Source: three-view drawing plus pictorial views. Frame: mm from the lowest corner of the part. Round coordinates to 2 decimals unless told otherwise and drop trailing zeros. Loops run counter-clockwise (first coordinate to the right, second up) from the corner with the lowest first, then second, coordinate; pieces in that order, holes last. Notation, with made-up numbers: M 73,-12 L 124,-12 A21 ccw 124,25 Z; hole C -37.5,56 d2. An arc over 180 degrees is marked long. Answer as a JSON object with one key per item and string values.
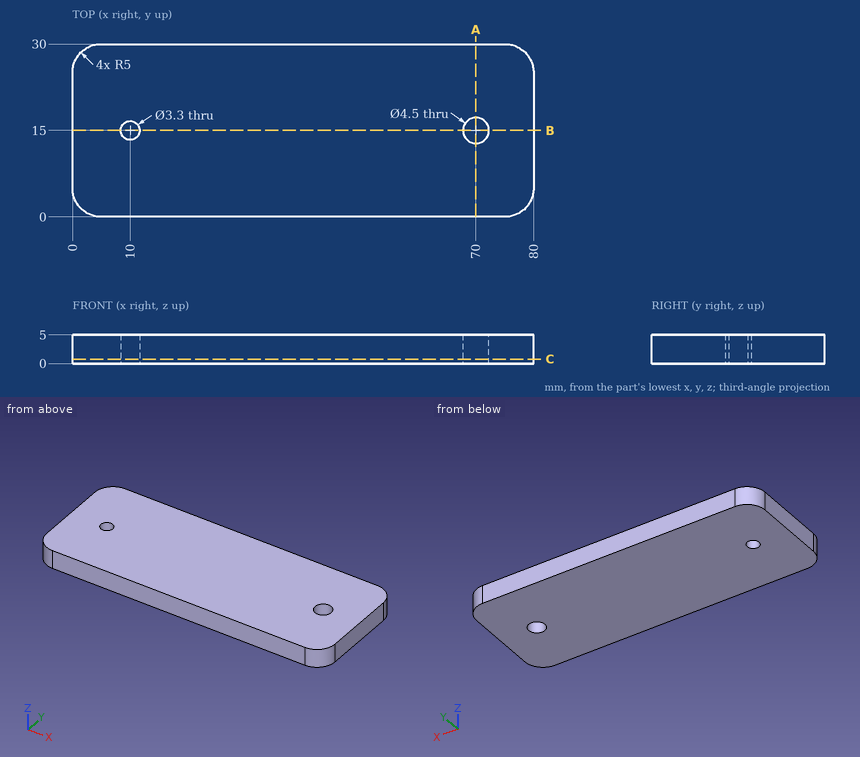
1) Line query: probe 1 along Y at (x, z) = (70, 1.6); probe 2 along Y at (x, z) = (10, 2.7); probe 3 along X at (y, z) = (16.25, 1.6). Output: solid intervals per line, ascending.
Geometry results:
{"probe 1": "0 to 12.75, 17.25 to 30", "probe 2": "0 to 13.35, 16.65 to 30", "probe 3": "0 to 8.92, 11.08 to 68.13, 71.87 to 80"}
2) Cut plane A-A on x = 70. Return the cut outline in (y, z), and give its area (4 significant figures).
Geometry results:
{"outline": "M 0,0 L 12.75,0 L 12.75,5 L 0,5 Z; M 17.25,0 L 30,0 L 30,5 L 17.25,5 Z", "area": "127.5 mm2"}
3) Cut plane C-C on z = 0.8. Return the cut outline in (x, y).
Geometry results:
{"outline": "M 0,5 A5 ccw 5,0 L 75,0 A5 ccw 80,5 L 80,25 A5 ccw 75,30 L 5,30 A5 ccw 0,25 Z; hole C 10,15 d3.3; hole C 70,15 d4.5"}
4) First-contact query: pin 1 (2.5 mm diameter, centred on x = 10, y = 15, fed in from -Z). Flat tip, straight axial feed; report the tip coordinate or a pass-through.
Geometry results:
{"pin 1": "through"}
5) Cut plane B-B on y = 15. Return the cut outline in (x, z).
Geometry results:
{"outline": "M 0,0 L 8.35,0 L 8.35,5 L 0,5 Z; M 11.65,0 L 67.75,0 L 67.75,5 L 11.65,5 Z; M 72.25,0 L 80,0 L 80,5 L 72.25,5 Z"}
